from build123d import *

# Parameters (mm, degrees)
SKETCH1_R           = 63.5
BOSS_EXTRUDE1_DEPTH = 6.35
SKETCH2_R           = 3.96875
CUT_EXTRUDE1_DEPTH  = 7.35


with BuildPart() as part:
    # Sketch1 → Boss-Extrude1 (new body)
    with BuildSketch(Plane.XY):
        Circle(SKETCH1_R)
    extrude(amount=BOSS_EXTRUDE1_DEPTH)

    # Sketch2 → Cut-Extrude1 (cut, through all)
    with BuildSketch(Plane.XY.offset(6.35)):
        Circle(SKETCH2_R)
        with Locations((-8.980256121, 8.980256121)):
            Circle(SKETCH2_R)
        with Locations((8.980256121, -8.980256121)):
            Circle(SKETCH2_R)
        with Locations((8.980256121, 8.980256121)):
            Circle(SKETCH2_R)
        with Locations((-8.980256121, -8.980256121)):
            Circle(SKETCH2_R)
        with Locations((17.960512242, -17.960512242)):
            Circle(SKETCH2_R)
        with Locations((35.921024484, -35.921024484)):
            Circle(SKETCH2_R)
        with Locations((-17.960512242, 17.960512242)):
            Circle(SKETCH2_R)
        with Locations((-35.921024484, 35.921024484)):
            Circle(SKETCH2_R)
    extrude(amount=-CUT_EXTRUDE1_DEPTH, mode=Mode.SUBTRACT)


solid = part.part
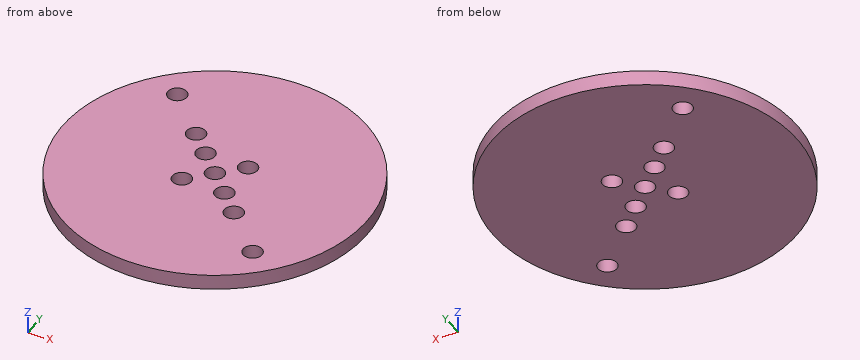
The listing builds one solid part. Answer for the finished solid, in the listing's coordinates (mm). Coordinates: 2 decimals unless noted, no trailing zeros. Loops run counter-clockwise (first coordinate to the right, second up) from the corner with the lowest first, then second, coordinate; pieces in that order, holes last.
1) Flat-ended cylindrical pins translate along their axes: pin 1 Ø5 at (x, y) = (8.98, -8.98) entering from -Z; pin 2 Ø1.5 at (x, z) = (-5.5, 5.5) entering from -Y; pin 3 Ø2 at (x, z) = (34.5, 1.5) entering from +Y; pin 4 Ø3 at (y, z) = (-9.5, 2) entering from -X. Find the tip coordinate at first contact, or state that the pin passes through.
2) Find section C-C on z = 4. Give the number of separate pieces and of enclosed holes in the cut face, then the cut area to 3 significant figures.
3) Find section D-D on x = 51.5. Write down the section's boundary in (y, z), then the cut area to 3 significant figures.
4) Find section A-A on y = 0. Write down the section's boundary in (x, z), then the cut area to 3 significant figures.
5) Find the intervals of material crossed by L1, parallel to Y at x = 0, z = 3.75; L2, parallel to X at y = -8, z = 4.75, in increasing order.
Values:
1. pin 1: passes through
1. pin 2: stops at y = -63.32
1. pin 3: stops at y = 53.94
1. pin 4: stops at x = -62.99
2. separate pieces: 1
2. enclosed holes: 9
2. area: 12,200 mm2
3. outline: (-37.15, 0) - (37.15, 0) - (37.15, 6.35) - (-37.15, 6.35) - close
3. area: 472 mm2
4. outline: (-63.5, 0) - (-3.97, 0) - (-3.97, 6.35) - (-63.5, 6.35) - close; (3.97, 0) - (63.5, 0) - (63.5, 6.35) - (3.97, 6.35) - close
4. area: 756 mm2
5. L1: y = -63.5 to -3.97, 3.97 to 63.5
5. L2: x = -62.99 to -12.83, -5.13 to 5.13, 12.83 to 62.99
